from build123d import *

# Parameters (mm, degrees)
BOSS_EXTRUDE1_DEPTH = 3.175
SKETCH2_R           = 2.55
CUT_EXTRUDE1_DEPTH  = 4.175
BOSS_EXTRUDE2_DEPTH = 3.175


with BuildPart() as part:
    # Sketch1 → Boss-Extrude1 (new body)
    with BuildSketch(Plane.XY):
        with BuildLine():
            Line((1.27, 12.636340451), (0, 15.176340451))
            Line((0, 15.176340451), (-1.27, 12.636340451))
            ThreePointArc((-1.27, 12.636340451), (-1.327511483, 12.630428071), (-1.384995456, 12.624253942))
            Line((-1.384995456, 12.624253942), (-3.155338604, 14.844701))
            Line((-3.155338604, 14.844701), (-3.869490362, 12.096158247))
            ThreePointArc((-3.869490362, 12.096158247), (-3.924515829, 12.078417757), (-3.979459965, 12.060426957))
            Line((-3.979459965, 12.060426957), (-6.172773769, 13.864276883))
            Line((-6.172773769, 13.864276883), (-6.299865427, 11.027315884))
            ThreePointArc((-6.299865427, 11.027315884), (-6.35, 10.998522628), (-6.400002977, 10.969501442))
            Line((-6.400002977, 10.969501442), (-8.920429101, 12.277917337))
            Line((-8.920429101, 12.277917337), (-8.454906143, 9.476526901))
            ThreePointArc((-8.454906143, 9.476526901), (-8.497958701, 9.437939284), (-8.540835149, 9.399156077))
            Line((-8.540835149, 9.399156077), (-11.278218876, 10.154953888))
            Line((-11.278218876, 10.154953888), (-10.240426889, 7.51156822))
            ThreePointArc((-10.240426889, 7.51156822), (-10.274515829, 7.464872704), (-10.308391842, 7.418022488))
            Line((-10.308391842, 7.418022488), (-13.143096367, 7.588170226))
            Line((-13.143096367, 7.588170226), (-11.578391842, 5.218317963))
            ThreePointArc((-11.578391842, 5.218317963), (-11.602027312, 5.165555367), (-11.625422345, 5.112685722))
            Line((-11.625422345, 5.112685722), (-14.43355748, 4.689747112))
            Line((-14.43355748, 4.689747112), (-12.410325511, 2.69700217))
            ThreePointArc((-12.410325511, 2.69700217), (-12.422474529, 2.640478473), (-12.434366108, 2.583900056))
            Line((-12.434366108, 2.583900056), (-15.09320287, 1.586359545))
            Line((-15.09320287, 1.586359545), (-12.699868404, 0.057814442))
            ThreePointArc((-12.699868404, 0.057814442), (-12.7, 0), (-12.699868404, -0.057814442))
            Line((-12.699868404, -0.057814442), (-15.09320287, -1.586359545))
            Line((-15.09320287, -1.586359545), (-12.434366108, -2.583900056))
            ThreePointArc((-12.434366108, -2.583900056), (-12.422474529, -2.640478473), (-12.410325511, -2.69700217))
            Line((-12.410325511, -2.69700217), (-14.43355748, -4.689747112))
            Line((-14.43355748, -4.689747112), (-11.625422345, -5.112685722))
            ThreePointArc((-11.625422345, -5.112685722), (-11.602027312, -5.165555367), (-11.578391842, -5.218317963))
            Line((-11.578391842, -5.218317963), (-13.143096367, -7.588170226))
            Line((-13.143096367, -7.588170226), (-10.308391842, -7.418022488))
            ThreePointArc((-10.308391842, -7.418022488), (-10.274515829, -7.464872704), (-10.240426889, -7.51156822))
            Line((-10.240426889, -7.51156822), (-11.278218876, -10.154953888))
            Line((-11.278218876, -10.154953888), (-8.540835149, -9.399156077))
            ThreePointArc((-8.540835149, -9.399156077), (-8.497958701, -9.437939284), (-8.454906143, -9.476526901))
            Line((-8.454906143, -9.476526901), (-8.920429101, -12.277917337))
            Line((-8.920429101, -12.277917337), (-6.400002977, -10.969501442))
            ThreePointArc((-6.400002977, -10.969501442), (-6.35, -10.998522628), (-6.299865427, -11.027315884))
            Line((-6.299865427, -11.027315884), (-6.172773769, -13.864276883))
            Line((-6.172773769, -13.864276883), (-3.979459965, -12.060426957))
            ThreePointArc((-3.979459965, -12.060426957), (-3.924515829, -12.078417757), (-3.869490362, -12.096158247))
            Line((-3.869490362, -12.096158247), (-3.155338604, -14.844701))
            Line((-3.155338604, -14.844701), (-1.384995456, -12.624253942))
            ThreePointArc((-1.384995456, -12.624253942), (-1.327511483, -12.630428071), (-1.27, -12.636340451))
            Line((-1.27, -12.636340451), (0, -15.176340451))
            Line((0, -15.176340451), (1.27, -12.636340451))
            ThreePointArc((1.27, -12.636340451), (1.327511483, -12.630428071), (1.384995456, -12.624253942))
            Line((1.384995456, -12.624253942), (3.155338604, -14.844701))
            Line((3.155338604, -14.844701), (3.869490362, -12.096158247))
            ThreePointArc((3.869490362, -12.096158247), (3.924515829, -12.078417757), (3.979459965, -12.060426957))
            Line((3.979459965, -12.060426957), (6.172773769, -13.864276883))
            Line((6.172773769, -13.864276883), (6.299865427, -11.027315884))
            ThreePointArc((6.299865427, -11.027315884), (6.35, -10.998522628), (6.400002977, -10.969501442))
            Line((6.400002977, -10.969501442), (8.920429101, -12.277917337))
            Line((8.920429101, -12.277917337), (8.454906143, -9.476526901))
            ThreePointArc((8.454906143, -9.476526901), (8.497958701, -9.437939284), (8.540835149, -9.399156077))
            Line((8.540835149, -9.399156077), (11.278218876, -10.154953888))
            Line((11.278218876, -10.154953888), (10.240426889, -7.51156822))
            ThreePointArc((10.240426889, -7.51156822), (10.274515829, -7.464872704), (10.308391842, -7.418022488))
            Line((10.308391842, -7.418022488), (13.143096367, -7.588170226))
            Line((13.143096367, -7.588170226), (11.578391842, -5.218317963))
            ThreePointArc((11.578391842, -5.218317963), (11.602027312, -5.165555367), (11.625422345, -5.112685722))
            Line((11.625422345, -5.112685722), (14.43355748, -4.689747112))
            Line((14.43355748, -4.689747112), (12.410325511, -2.69700217))
            ThreePointArc((12.410325511, -2.69700217), (12.422474529, -2.640478473), (12.434366108, -2.583900056))
            Line((12.434366108, -2.583900056), (15.09320287, -1.586359545))
            Line((15.09320287, -1.586359545), (12.699868404, -0.057814442))
            ThreePointArc((12.699868404, -0.057814442), (12.7, 0), (12.699868404, 0.057814442))
            Line((12.699868404, 0.057814442), (15.09320287, 1.586359545))
            Line((15.09320287, 1.586359545), (12.434366108, 2.583900056))
            ThreePointArc((12.434366108, 2.583900056), (12.422474529, 2.640478473), (12.410325511, 2.69700217))
            Line((12.410325511, 2.69700217), (14.43355748, 4.689747112))
            Line((14.43355748, 4.689747112), (11.625422345, 5.112685722))
            ThreePointArc((11.625422345, 5.112685722), (11.602027312, 5.165555367), (11.578391842, 5.218317963))
            Line((11.578391842, 5.218317963), (13.143096367, 7.588170226))
            Line((13.143096367, 7.588170226), (10.308391842, 7.418022488))
            ThreePointArc((10.308391842, 7.418022488), (10.274515829, 7.464872704), (10.240426889, 7.51156822))
            Line((10.240426889, 7.51156822), (11.278218876, 10.154953888))
            Line((11.278218876, 10.154953888), (8.540835149, 9.399156077))
            ThreePointArc((8.540835149, 9.399156077), (8.497958701, 9.437939284), (8.454906143, 9.476526901))
            Line((8.454906143, 9.476526901), (8.920429101, 12.277917337))
            Line((8.920429101, 12.277917337), (6.400002977, 10.969501442))
            ThreePointArc((6.400002977, 10.969501442), (6.35, 10.998522628), (6.299865427, 11.027315884))
            Line((6.299865427, 11.027315884), (6.172773769, 13.864276883))
            Line((6.172773769, 13.864276883), (3.979459965, 12.060426957))
            ThreePointArc((3.979459965, 12.060426957), (3.924515829, 12.078417757), (3.869490362, 12.096158247))
            Line((3.869490362, 12.096158247), (3.155338604, 14.844701))
            Line((3.155338604, 14.844701), (1.384995456, 12.624253942))
            ThreePointArc((1.384995456, 12.624253942), (1.327511483, 12.630428071), (1.27, 12.636340451))
        make_face()
    extrude(amount=BOSS_EXTRUDE1_DEPTH)

    # Sketch2 → Cut-Extrude1 (cut, through all)
    with BuildSketch(Plane.XY.offset(3.175)):
        Circle(SKETCH2_R)
    extrude(amount=-CUT_EXTRUDE1_DEPTH, mode=Mode.SUBTRACT)

    # Sketch3 → Boss-Extrude2 (add, through all)
    with BuildSketch(Plane.XY.offset(3.175)):
        with BuildLine():
            Line((-1.27, 2.211243994), (1.27, 2.211243994))
            ThreePointArc((1.27, 2.211243994), (0, 2.55), (-1.27, 2.211243994))
        make_face()
    extrude(amount=-BOSS_EXTRUDE2_DEPTH)


solid = part.part
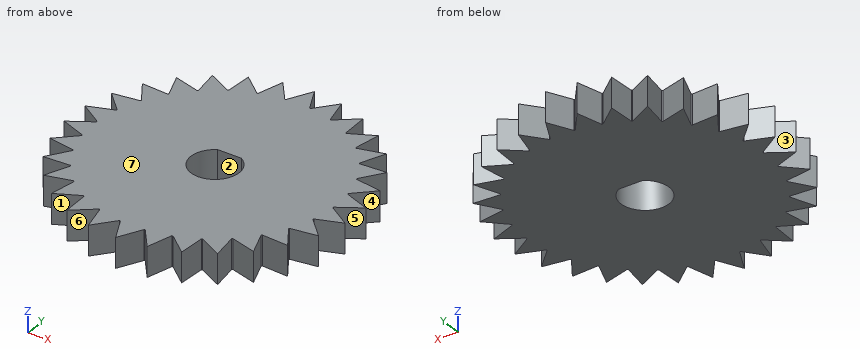
Design review of the part built by this model. Coordinates are the model's own, in mm. Face numbers are marked on the shaded views. A direction names the side the tool comes from. Coordinates: 2 decimals unless noted, no trailing zeros. Loops run counter-clockwise (first coordinate to the right, second up) from the corner with the lowest first, then second, coordinate; pieces in that order, holes last.
Item 1: Clearance check with flat-ended pins moving along their axes: pin 1 (0.8 mm diameter, centred on x = 0.5, z = 2, fed in from -Y); pin 2 (1 mm diameter, centred on x = 11.5, z = 2, fed in from +Y). State where each tip first meets the part, or that it passes through.
Completed:
pin 1: stops at y = -14.98
pin 2: stops at y = 10.15
Item 2: Add section D-D (y = -9). Write out the cut boundary in (x, z) (3 decimals), and give its area (3 significant figures).
Completed:
outline: (-10.825, 0) - (10.825, 0) - (10.825, 3.175) - (-10.825, 3.175) - close
area: 68.7 mm2
Item 3: Add section A-A (x = -12). Write out the cut boundary in (y, z) (3 decimals), and give its area (3 significant figures).
Completed:
outline: (-7.52, 0) - (-5.857, 0) - (-5.857, 3.175) - (-7.52, 3.175) - close; (-5.056, 0) - (5.056, 0) - (5.056, 3.175) - (-5.056, 3.175) - close; (5.857, 0) - (7.52, 0) - (7.52, 3.175) - (5.857, 3.175) - close
area: 42.7 mm2
Item 4: Wall thickness on L1, parallel to X at y = 0, z = 2.05; L2, parallel to X at y = -12, z = 2.4; L3, parallel to Y at x = -12, z = 2.6: over which ranges is each line inside the solid? List them lowest first.
Completed:
L1: x = -12.7 to -2.55, 2.55 to 12.7
L2: x = -8.87 to -8.39, -6.26 to 6.26, 8.39 to 8.87
L3: y = -7.52 to -5.86, -5.06 to 5.06, 5.86 to 7.52
Item 5: Add section C-C (x = 13.5). Write out the cut boundary in (y, z) (3 decimals).
Completed:
outline: (-4.83, 0) - (-3.77, 0) - (-3.77, 3.175) - (-4.83, 3.175) - close; (-2.184, 0) - (-0.569, 0) - (-0.569, 3.175) - (-2.184, 3.175) - close; (0.569, 0) - (2.184, 0) - (2.184, 3.175) - (0.569, 3.175) - close; (3.77, 0) - (4.83, 0) - (4.83, 3.175) - (3.77, 3.175) - close
Item 6: For the marked faces 1, 2, 3 and 4, list the 3-axis set-ups (+Z, -Z, +X, -X, +Y, -Y) from which the entire face can be reached by the end or side of a thin tool; tool diameter is ignored.
Completed:
face 1: +Z, -Z, -Y
face 2: +Z, -Z
face 3: +Z, -Z, -X
face 4: +Z, -Z, +X
Item 7: Add section B-B (x = -0.5). Write out the cut boundary in (y, z) (1 decimal).
Completed:
outline: (-14.2, 0) - (-2.5, 0) - (-2.5, 3.2) - (-14.2, 3.2) - close; (2.2, 0) - (14.2, 0) - (14.2, 3.2) - (2.2, 3.2) - close
Item 8: Draft analysis for pull direction X (two halves, no side actions). For the marked faces 5, 6 and 7, state which applies: pulls with the +X half, pulls with the -X half, needs draft (parallel to the pull), parting line crosses it, or undercut.
Completed:
face 5: pulls with the +X half
face 6: undercut
face 7: needs draft
